Could you check a few things on this model? Use its own coordinates, in mm. A direction names the side the tool comes from. Give positions to 0.01 mm unless a question says otherwise; leave off trailing zeros. Write each loop counter-clockwise with the first axis right and the second up, starting at its lowest first coordinate (ties: lowest second). Pieces come first, ordered by that corner, then holes. Notation, with made-up numbers: (34, 30.25) - (45, 30.25) arc R17 cw to (45, 60.25) - close; hole circle Ø11 at (70.5, 74). An arc over 180 degrees is marked (long way). Answer as CSV lines item,"result". Start each with the question number.
Q1. Imagine slicing it at A-A on x = 7.25. List the corners of the cut face in (y, z) for me, and give its area (3 significant figures).
Q2. We'd pull the mould along Z, two halves only. Please class faces 4 (the face through (10, 0, 0)), 5 (the face through (-3.77, -1.74, -0.99)), 6 (the face through (-2.218, 2.285, 3.584)), 7 (the face through (-1.998, -0.122, -0.027)): pulls with the +Z half, pulls with the -Z half, needs draft (parallel to the pull), parting line crosses it, or undercut.
Q3. Will these pins go through, and if not, where does the flat tip stop? pin 1 Ø5 at (x, z) = (-0.5, 3) entering from +Y; pin 2 Ø3 at (x, z) = (7, -3) entering from -Y; pin 3 Ø2 at (x, y) = (5, 1) entering from -Z.
Q4. On a 3-axis mill with a long thin cutter (end or side, diameter ignored), from which of +Z, -Z, +X, -X, +Y, -Y can I reach the whole of each face in a straight line? I mean faces 1 (the face through (0, 2, -2)), 2 (the face through (-3.768, -1.724, 1.014)), 3 (the face through (-5, 2, -2)). Say none if no direction works.
Q5. If I drill on line 1 along X through (y, z) = (2.5, -2); line 2 along Z through (x, y) = (-2, -2); line 3 along Y through (x, z) = (0.75, 1.5), over which ranges is the centre line in solid material (lowest first)?
Autodesk Inventor part; units mm, degrees
ref_plane "bolt_to_nut_XY" through (10, 0, 0) normal (1, 0, 0) x (0, 0, -1)
ref_plane "bolt_to_nut_YZ" through (10, 0, 0) normal (0, 0, -1) x (0, 1, 0)
ref_plane "bolt_to_nut_ZX" through (10, 0, 0) normal (0, 1, 0) x (1, 0, 0)
sketch "Sketch_1" plane through (0, 0, 0) normal (0, 0, 1) x (1, 0, 0)
  line L0 (10, 0) -> (-5, 0)
  line L1 (-5, 0) -> (-5, 3.75)
  line L2 (-5, 3.75) -> (-4.5, 4.25)
  line L3 (-4.5, 4.25) -> (0, 4.25)
  line L4 (0, 4.25) -> (0, 2.5)
  line L5 (0, 2.5) -> (9.5095, 2.5)
  line L6 (9.5095, 2.5) -> (10, 2.0095)
  line L7 (10, 2.0095) -> (10, 0)
  line L8 (10, 0) -> (-5, 0)
revolve "Revolution1" add sketch "Sketch_1" angle 360 about axis through (10, 0, 0) along (1, 0, 0)
thread "Thread1"
sketch "Sketch2" plane through (-5, 0, 0) normal (-1, 0, 0) x (0, 0, 1)
  point P0 (0, 0)
hole "Hole1" at (-5, 0, 0) direction (1, 0, 0) diameter 4 depth 2.5 tip angle 150
sketch "Sketch_3" plane through (-5, 0, 0) normal (1, 0, 0) x (0, 0, -1)
  line L0 (-2, 1.1547) -> (-2, -1.1547)
  line L1 (-2, -1.1547) -> (0, -2.3094)
  line L2 (0, -2.3094) -> (2, -1.1547)
  line L3 (2, -1.1547) -> (2, 1.1547)
  line L4 (2, 1.1547) -> (0, 2.3094)
  line L5 (0, 2.3094) -> (-2, 1.1547)
extrude "Extrusion1" cut sketch "Sketch_3" along normal blind 2.5
ref_plane "bolt_to_nut_XY" through (10, 0, 0) normal (1, 0, 0) x (0, 0, -1)
ref_plane "bolt_to_nut_YZ" through (10, 0, 0) normal (0, 0, -1) x (0, 1, 0)
ref_plane "bolt_to_nut_ZX" through (10, 0, 0) normal (0, 1, 0) x (1, 0, 0)
ref_plane "screw1_XY" through (0, 0, 0) normal (1, 0, 0) x (0, 0, -1)
ref_plane "screw1_YZ" through (0, 0, 0) normal (0, 0, -1) x (0, 1, 0)
ref_plane "screw1_ZX" through (0, 0, 0) normal (0, 1, 0) x (1, 0, 0)
properties part number "CB5-10" material "鋼、炭素鋼"
Conclusion:
1,outline,"circle Ø5 at (0, 0)"
1,area,"19.6 mm^2"
2,face 4,"needs draft"
2,face 5,"undercut"
2,face 6,"parting line crosses it"
2,face 7,"undercut"
3,pin 1,"y = 4.22"
3,pin 2,"y = -2"
3,pin 3,"z = -2.5"
4,face 1,"+X"
4,face 2,"-X"
4,face 3,"+Z, -Z, -X, +Y, -Y"
5,line 1,"-5 to 0"
5,line 2,"-3.75 to 3.75"
5,line 3,"-2 to 2"
